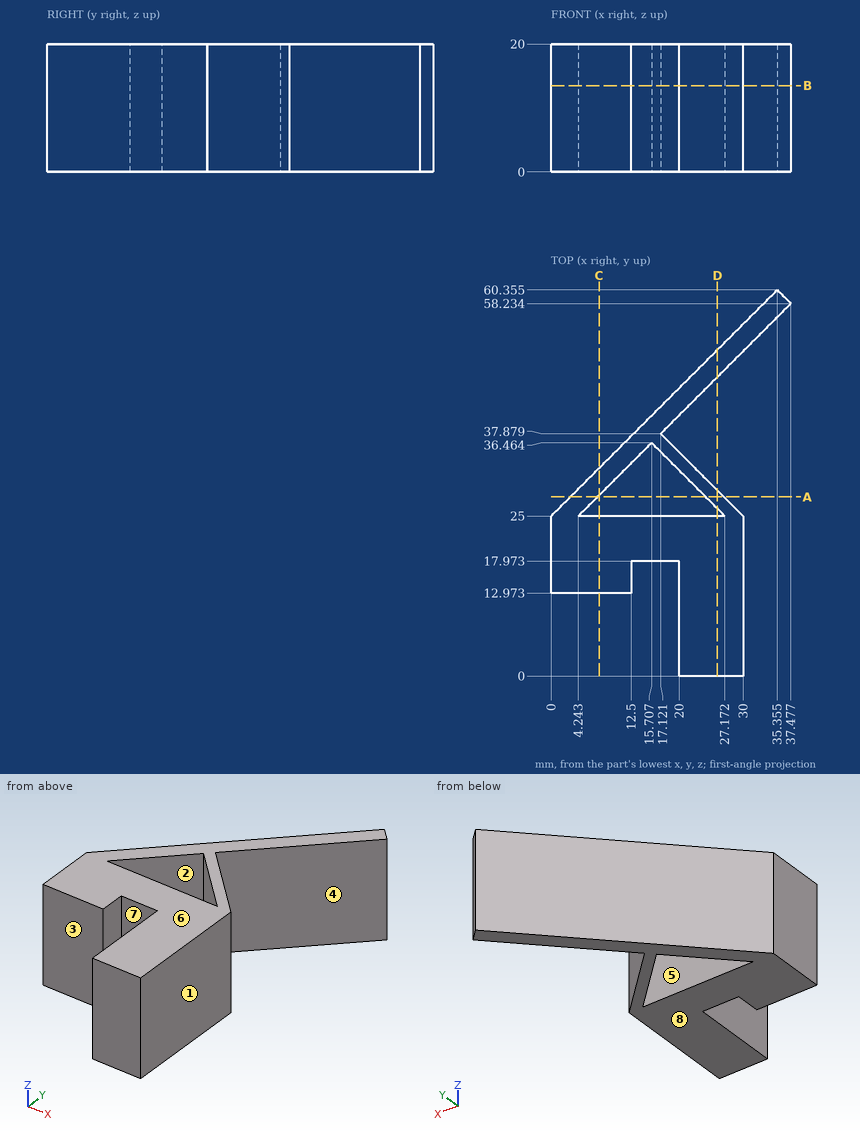
Drawing for the job (mm, zero at the part's lowest x, y, z). A direction names the side the tool comes from. Give positions to 0.01 mm unless a question says otherwise; leave off trailing zeros. Order: outer loops, then holes, each group sorted by start corner. A loop starts at its lowest first (then second) coordinate and runs counter-clockwise, first axis right, second up. Notation, with made-up numbers: (43, 74.25) -> (69, 74.25) arc R18 cw to (69, 83.25) -> close; hole circle Ø10 at (-36, -2). An arc over 180 degrees is marked (long way). Use one line per item in the form item = value.
(1) Pull direction X, two halves, no side cores. Call the marked faces 1, 2 and 3: +X half, -X half, draft (parallel to the pull), parting line (faces both ways), or undercut.
Solution:
face_1 = +X half
face_2 = undercut
face_3 = draft
(2) Saw through at A-A (y = 28). Write the cut outline in (x, z).
Solution:
outline = (3, 0) -> (7.24, 0) -> (7.24, 20) -> (3, 20) -> close; (24.17, 0) -> (27, 0) -> (27, 20) -> (24.17, 20) -> close
(3) Drill centre lines: line 1 (X direction, y = 16, z = 8.5); line 2 (Y direction, x = 25, z = 1.75) (1 decimal); line 3 (X direction, y = 23, z = 7.25). Where is each one in solid material? Low to high. Write a range as from..to.
Solution:
line_1 = 0..12.5, 20..30
line_2 = 0..25, 27.2..30, 45.8..50
line_3 = 0..30
(4) Tool access for the marked faces 4, 5, 6, 7 and 8: list every direction of +Z, -Z, +X, -X, +Y, -Y with a clear straight run to the whole face (end or side of a thin tool).
Solution:
face_4 = +Z, -Z, +X
face_5 = +Z, -Z
face_6 = +Z, +X, -X, +Y, -Y
face_7 = +Z, -Z, -Y
face_8 = -Z, +X, -X, +Y, -Y
(5) Saw through at B-B (z = 13.5). Write the cut outline in (x, y) (1 decimal).
Solution:
outline = (0, 13) -> (12.5, 13) -> (12.5, 18) -> (20, 18) -> (20, 0) -> (30, 0) -> (30, 25) -> (17.1, 37.9) -> (37.5, 58.2) -> (35.4, 60.4) -> (0, 25) -> close; hole (4.2, 25) -> (27.2, 25) -> (15.7, 36.5) -> close
(6) Flat gauge pins, fed straight in: P1, Ø1.5, axis at y = 17, z = 18, coming from the +X side; P2, Ø1.5, axis at x = 6, z = 4, coming from the +Y side; P3, Ø9, axis at y = 6, z = 11, coming from the -X side; P4, Ø8, axis at x = 14.5, y = 35, coming from the +Z side. Where does each tip first touch, or does it go through?
Solution:
P1 = 30
P2 = 31.75
P3 = 20
P4 = 20
(7) Saw through at C-C (x = 7.5). Write the cut outline in (y, z), then the cut area to 3 significant figures.
Solution:
outline = (12.97, 0) -> (25, 0) -> (25, 20) -> (12.97, 20) -> close; (28.26, 0) -> (32.5, 0) -> (32.5, 20) -> (28.26, 20) -> close
area = 325 mm²
(8) Saw through at D-D (x = 26). Write the cut outline in (y, z).
Solution:
outline = (0, 0) -> (25, 0) -> (25, 20) -> (0, 20) -> close; (26.17, 0) -> (29, 0) -> (29, 20) -> (26.17, 20) -> close; (46.76, 0) -> (51, 0) -> (51, 20) -> (46.76, 20) -> close
